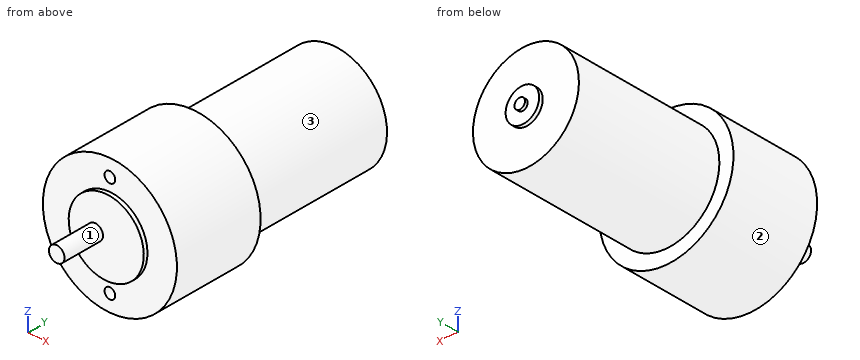
```python
from build123d import *

# Parameters (mm, degrees)
SKETCH1_R                  = 25.4
BOSS_EXTRUDE1_DEPTH        = 34.798
SKETCH2_R                  = 20.066
BOSS_EXTRUDE2_DEPTH        = 58.42
SKETCH3_R                  = 14.224
BOSS_EXTRUDE3_DEPTH        = 1.524
SKETCH4_R                  = 6.35
BOSS_EXTRUDE4_DEPTH        = 1.4732
SKETCH5_R                  = 1.9812
BOSS_EXTRUDE5_DEPTH        = 1.1176
SKETCH6_R                  = 2.9464
BOSS_EXTRUDE6_DEPTH        = 17.526
F_10_32_TAPPED_HOLE1_D     = 4.0386
F_10_32_TAPPED_HOLE1_DEPTH = 6.35
F_10_32_TAPPED_HOLE1_TIP   = 1.213317848


with BuildPart() as part:
    # Sketch1 → Boss-Extrude1 (new body)
    with BuildSketch(Plane(origin=(0, 0, 0), x_dir=(1, 0, 0), z_dir=(0, 1, 0))):
        with Locations(Location((0, 0, 0), (0, 0, 270))):
            Circle(SKETCH1_R)
    extrude(amount=BOSS_EXTRUDE1_DEPTH)

    # Sketch2 → Boss-Extrude2 (add)
    with BuildSketch(Plane(origin=(0, 34.798, 0), x_dir=(-1, 0, 0), z_dir=(0, 1, 0))):
        with Locations(Location((0, 0, 0), (0, 0, 270))):
            Circle(SKETCH2_R)
    extrude(amount=BOSS_EXTRUDE2_DEPTH)

    # Sketch3 → Boss-Extrude3 (add)
    with BuildSketch(Plane.XZ):
        with Locations(Location((0, 0, 0), (0, 0, 90))):
            Circle(SKETCH3_R)
    extrude(amount=BOSS_EXTRUDE3_DEPTH)

    # Sketch4 → Boss-Extrude4 (add)
    with BuildSketch(Plane(origin=(0, 93.218, 0), x_dir=(-1, 0, 0), z_dir=(0, 1, 0))):
        with Locations(Location((0, 0, 0), (0, 0, 90))):
            Circle(SKETCH4_R)
    extrude(amount=BOSS_EXTRUDE4_DEPTH)

    # Sketch5 → Boss-Extrude5 (add)
    with BuildSketch(Plane(origin=(0, 94.6912, 0), x_dir=(1, 0, 0), z_dir=(0, 1, 0))):
        with Locations(Location((0, 0, 0), (0, 0, 270))):
            Circle(SKETCH5_R)
    extrude(amount=BOSS_EXTRUDE5_DEPTH)

    # Sketch6 → Boss-Extrude6 (add)
    with BuildSketch(Plane.XZ):
        with Locations(Location((-4.1783, 0, 0), (0, 0, 270))):
            Circle(SKETCH6_R)
    extrude(amount=BOSS_EXTRUDE6_DEPTH)

    # #10-32 Tapped Hole1
    with Locations(Plane.XZ):
        with Locations((0, 19.05), (0, -19.05)):
            Hole(F_10_32_TAPPED_HOLE1_D / 2, depth=F_10_32_TAPPED_HOLE1_DEPTH)
            with Locations((0, 0, -(F_10_32_TAPPED_HOLE1_DEPTH + F_10_32_TAPPED_HOLE1_TIP / 2))):  # 118° drill point
                Cone(0, F_10_32_TAPPED_HOLE1_D / 2, F_10_32_TAPPED_HOLE1_TIP, mode=Mode.SUBTRACT)


solid = part.part
```
Input: part model. Units: mm. Frame: model coordinates. Face numbers are marked on the shaded views. A direction names the side the tool comes from. Give positions to 0.01 mm unless a question says otherwise; leave off trailing zeros. Loops run counter-clockwise (first coordinate to the right, second up) from the corner with the lowest first, then second, coordinate; pieces in that order, holes last. Notation, with made-up numbers: M -7.75,-25.5 L 43.25,-25.5 A15 cw 43.25,-2.5 Z; hole C -33.5,70.25 d3. An arc over 180 degrees is marked long. Answer as CSV lines item,"result". Start each with the question number.
1. Pin query (flat end, axial travel): P1, Ø2, axis at y = 21.5, z = -4, coming from the +X side; P2, Ø4.5, axis at x = 0, z = -19.05, coming from the -Y side; P3, Ø4, axis at x = 3, z = -1.5, coming from the +Y side; P4, Ø4, axis at x = -8, y = 40.5, coming from the +Z side. Return the tip coordinate at first contact, or that it passes through.
2. Line query: L1, parallel to Z at x = -1, y = 45; L2, parallel to Y at x = 5, z = -2; L3, parallel to Y at x = 11.5, z = 12. Output: solid intervals per line, ascending.
3. Section B-B on x = -11. Return loops of the section in (y, z).
4. Section D-D on z = -12. Return loops of the section in (x, y), plus the area to 3 significant figures.
5. Section A-A on z = 0. Return loops of the section in (x, y).
6. Reachability of the marked faces 1, 2 and 3 from +Z, -Z, +X, -X, +Y, -Y: full face, straight path, thin tool, end or side. Return the list, or none.
7. Section C-C on y = 74. Return loops of the section in (x, z).
Computed values:
1,P1,"stops at x = 25.22"
1,P2,"stops at y = 0"
1,P3,"stops at y = 95.81"
1,P4,"stops at z = 19.15"
2,L1,"z = -20.04 to 20.04"
2,L2,"y = -1.52 to 94.69"
2,L3,"y = 0 to 93.22"
3,outline,"M -1.52,-9.02 L 0,-9.02 L 0,-22.89 L 34.8,-22.89 L 34.8,-16.78 L 93.22,-16.78 L 93.22,16.78 L 34.8,16.78 L 34.8,22.89 L 0,22.89 L 0,9.02 L -1.52,9.02 Z"
4,outline,"M -22.39,0 L -7.64,0 L -7.64,-1.52 L 7.64,-1.52 L 7.64,0 L 22.39,0 L 22.39,34.8 L 16.08,34.8 L 16.08,93.22 L -16.08,93.22 L -16.08,34.8 L -22.39,34.8 Z"
4,area,"3,460 mm²"
5,outline,"M -25.4,0 L -14.22,0 L -14.22,-1.52 L -7.12,-1.52 L -7.12,-17.53 L -1.23,-17.53 L -1.23,-1.52 L 14.22,-1.52 L 14.22,0 L 25.4,0 L 25.4,34.8 L 20.07,34.8 L 20.07,93.22 L 6.35,93.22 L 6.35,94.69 L 1.98,94.69 L 1.98,95.81 L -1.98,95.81 L -1.98,94.69 L -6.35,94.69 L -6.35,93.22 L -20.07,93.22 L -20.07,34.8 L -25.4,34.8 Z"
6,face 1,"-Y"
6,face 2,"+Y, -Y"
6,face 3,"+Y"
7,outline,"C 0,0 d40.13"
